Could you check a few things on this drawing? It's one solid part, dimensions in mm from its lowest x, y, z. A direction names the side the tool comes from. Give positions to 0.01 mm unless a question says otherwise; leave off trailing zeros. Loops run counter-clockwise (first coordinate to the right, second up) from the corner with the lowest first, then second, coordinate; pieces in that order, holes last.
1. Imagine slicing it at C-C (x = 10.75). Count the separate pieces of the cut face and the enclosed holes in it, plus the area to 3 significant figures.
2. I need wall thicknesses on line 1 along Y through (x, z) = (5, 4.2); line 2 along X through (y, z) = (17, 18); line 3 along Z through (x, y) = (12, 18.4). Which ranges of each line are inside material? Lowest first, please.
3. Thinking about a two-plate mould opening in X: for the marked faces 6, 7 and 8, which applies, +X half, -X half, draft (parallel to the pull), parting line (faces both ways), or undercut?
4. Imagine slicing it at B-B (y = 30). List the corners of the cut face in (x, z) for me, plus the area to 3 significant figures.
5. Imagine slicing it at A-A (z = 18). List the corners of the cut face in (x, y) for me.
6. For P1, Ø9.5, axis at x = 5, y = 5, coming from the +Z side; P2, Ø5, axis at x = 3, z = 19, coming from the +Y side; P3, Ø3, axis at y = 22, z = 12.5, coming from the +X side, each with a flat end and sliding along its axis, tell me the tip position at first contact or that it passes through.
7. For the marked faces 1, 2, 3, 4 and 5, which set-ups out of +Z, -Z, +X, -X, +Y, -Y let a thin tool reach every point of the face, with its end or its side?
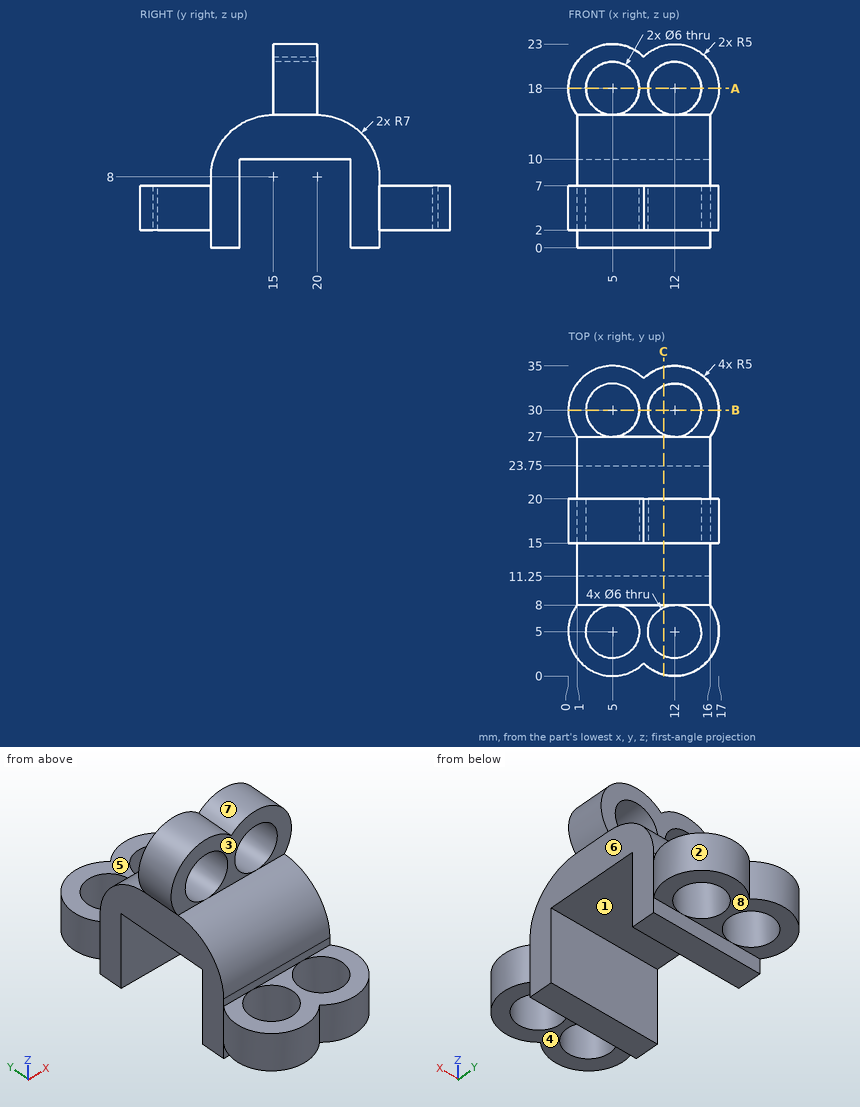
Derived:
1. separate pieces: 4
1. enclosed holes: 0
1. area: 175 mm2
2. line 1: y = 0 to 2, 8 to 11.25, 23.75 to 27, 33 to 35
2. line 2: x = 0 to 2, 8 to 9, 15 to 17
2. line 3: z = 10 to 15, 21 to 23
3. face 6: +X half
3. face 7: undercut
3. face 8: draft
4. outline: (0, 2) - (2, 2) - (2, 7) - (0, 7) - close; (8, 2) - (9, 2) - (9, 7) - (8, 7) - close; (15, 2) - (17, 2) - (17, 7) - (15, 7) - close
4. area: 25.0 mm2
5. outline: (0, 15) - (2, 15) - (2, 20) - (0, 20) - close; (8, 15) - (9, 15) - (9, 20) - (8, 20) - close; (15, 15) - (17, 15) - (17, 20) - (15, 20) - close
6. P1: stops at z = 12.63
6. P2: stops at y = 20
6. P3: stops at x = 16
7. face 1: -Z, +X, -X
7. face 2: +Z, -Z
7. face 3: +Z, +X, -X, -Y
7. face 4: -Z, +X, -X, -Y
7. face 5: +Z, +X, -X, +Y
